Geometry: final body of the model. Coordinates: model frame, mm. Face numbers are marked on the shaded views. A direction names the side the tool comes from. Round coordinates to 2 decimals unless told otherwise and drop trailing zeros. Loops run counter-clockwise (first coordinate to the right, second up) from the corner with the lowest first, then second, coordinate; pieces in that order, holes last. Notation, with made-up numbers: M 87,40 L 125,40 A21 ccw 125,49 Z; hole C -22,52 d7. An arc over 180 degrees is marked long. Answer as a JSON object with one key per item and string values.
from build123d import *

# Parameters (mm, degrees)
ESQUISSE2_R             = 2.5
BASE_EXTRUSION_DEPTH    = 16
CHANFREIN1_SIZE         = 0.5
ENL_V_MAT_EXTRU_1_DEPTH = 2.5


with BuildPart() as part:
    # Esquisse2 → Base-Extrusion (new body)
    with BuildSketch(Plane(origin=(0, 0, 0), x_dir=(1, 0, 0), z_dir=(0, 1, 0))):
        with Locations(Location((0, 0, 0), (0, 0, 270))):  # turned: the seam where the file's is
            Circle(ESQUISSE2_R)
    extrude(amount=-BASE_EXTRUSION_DEPTH)

    # Chanfrein1
    chanfrein1_edges = [part.edges().sort_by_distance(p)[0] for p in [
        (0, -16, -2.5),
    ]]
    chamfer(chanfrein1_edges, length=CHANFREIN1_SIZE)

    # Esquisse5 → Boss.-Révol.1 (revolve)
    with BuildSketch(Plane.XY, mode=Mode.PRIVATE) as boss_r_vol_1_sk:
        with BuildLine():
            Line((2, 5), (2, 2.5))
            Line((2, 2.5), (0, 1.345299462))
            Line((0, 1.345299462), (0, 0))
            Line((0, 0), (4.25, 0))
            Line((4.25, 0), (4.25, 4.5))
            ThreePointArc((4.25, 4.5), (4.103553391, 4.853553391), (3.75, 5))
            Line((3.75, 5), (2, 5))
        make_face()
    revolve(boss_r_vol_1_sk.sketch.rotate(Axis((0, 5, 0), (0, -1, 0)), 90), axis=Axis((0, 5, 0), (0, -1, 0)))  # turned: the seam where the file's is

    # Esquisse7 → Enlèv. mat.-Extru.1 (cut)
    with BuildSketch(Plane(origin=(0, 5, 0), x_dir=(-1, 0, 0), z_dir=(0, 1, 0))):
        Polygon((1.154700538, 2), (-1.154700538, 2), (-2.309401077, 0), (-1.154700538, -2), (1.154700538, -2), (2.309401077, 0), align=None)
    extrude(amount=-ENL_V_MAT_EXTRU_1_DEPTH, mode=Mode.SUBTRACT)


solid = part.part
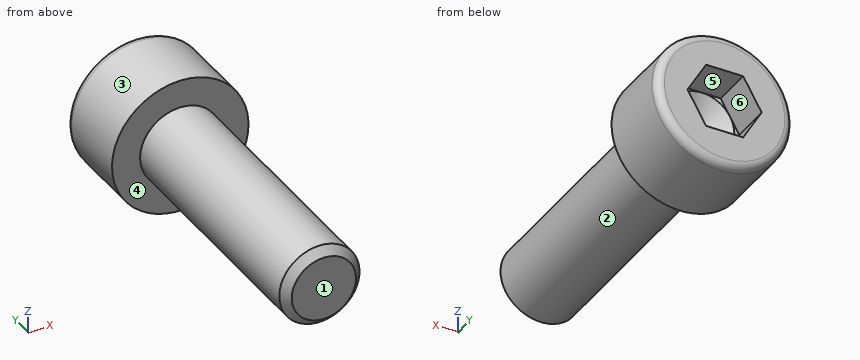
1) Section query B-B (y = 0.5). Return the cut outline in (x, z).
Results:
{"outline": "C 0,0 d8.5"}
2) Reachability of the marked faces 1 and 2 from +Z, -Z, +X, -X, +Y, -Y: full face, straight path, thin tool, end or side. Return the list, or none.
Results:
{"face 1": "+Z, -Z, +X, -X, -Y", "face 2": "-Y"}
3) Section query A-A (y = 2.75). Return the cut outline in (x, z).
Results:
{"outline": "C 0,0 d8.5; hole M -2.31,0 L -1.15,-2 L 1.15,-2 L 2.31,0 L 1.15,2 L -1.15,2 Z"}
4) Pull-direction query (X, two-part tool) for the marked faces 3, 4, 5 and 6; classes: +X half, -X half, draft (parallel to the pull), parting line (faces both ways), or undercut.
Results:
{"face 3": "parting line", "face 4": "draft", "face 5": "undercut", "face 6": "undercut"}
5) Ray query, line 1 (Y direction, x = 2.25, z = -2.75); line 2 (X direction, y = -8.75, z = -1.5). Return the intervals inside material, ascending.
Results:
{"line 1": "0 to 5", "line 2": "-2 to 2"}
6) Pin query (flat end, axial travel): P1, Ø0.5, axis at x = 0.5, z = 1.5, coming from the +Y side; P2, Ø5, axis at y = -7.5, z = 1, coming from the -X side; P3, Ø2, axis at y = -12.5, z = 2.5, coming from the +X side. Return the tip coordinate at first contact, or that it passes through.
Results:
{"P1": "y = 2.4", "P2": "x = -2.5", "P3": "x = 2"}
7) Section query C-C (y = -7). Return the cut outline in (x, z).
Results:
{"outline": "C 0,0 d5"}
